```python
from build123d import *

# Parameters (mm, degrees)
BOSS_EXTRUDE1_DEPTH = 12
SKETCH2_R           = 5.25
CUT_EXTRUDE1_DEPTH  = 6
CHAMFER2_SIZE       = 3
CHAMFER2_SIZE2      = 5.196152423
SKETCH4_R           = 2.75
CUT_EXTRUDE3_DEPTH  = 28
CUT_EXTRUDE4_REACH  = 38.986
SKETCH5_W           = 8.2
SKETCH5_H           = 5.3
CUT_EXTRUDE6_REACH  = 38.986
CHAMFER3_SIZE       = 5
SKETCH8_R           = 2.95
BOSS_EXTRUDE2_DEPTH = 5
CHAMFER4_SIZE       = 5
CHAMFER4_SIZE2      = 10.722534603


with BuildPart() as part:
    # Sketch1 → Boss-Extrude1 (new, symmetric)
    with BuildSketch(Plane.XY):
        Polygon((-9, 8), (4, 8), (4, -30), (-14, -30), (-14, 0), (-3, 0), (-3, 4), (-9, 4), align=None)
    extrude(amount=BOSS_EXTRUDE1_DEPTH, both=True)

    # Sketch2 → Cut-Extrude1 (cut)
    with BuildSketch(Plane.XZ.offset(30)):
        with Locations((-5, 0)):
            Circle(SKETCH2_R)
    extrude(amount=-CUT_EXTRUDE1_DEPTH, mode=Mode.SUBTRACT)

    # Chamfer2
    chamfer2_edges = [part.edges().sort_by_distance(p)[0] for p in [
        (-14, 0, 0),
    ]]
    chamfer2_side = [part.faces().sort_by_distance(p)[0] for p in [
        (-8.5, 0, 0),
    ]]
    chamfer(chamfer2_edges, length=CHAMFER2_SIZE, length2=CHAMFER2_SIZE2, reference=chamfer2_side[0])

    # Sketch4 → Cut-Extrude3 (cut)
    with BuildSketch(Plane.XZ.offset(30)):
        with Locations((-5, 0)):
            Circle(SKETCH4_R)
    extrude(amount=-CUT_EXTRUDE3_DEPTH, mode=Mode.SUBTRACT)

    # Sketch5 → Cut-Extrude4 (cut, up to next)
    with BuildSketch(Plane(origin=(4, 0, 0), x_dir=(0, 0, -1), z_dir=(1, 0, 0)), mode=Mode.PRIVATE) as cut_extrude4_sk1:
        with Locations((0, -16.65)):
            Rectangle(SKETCH5_W, SKETCH5_H)
    cut_extrude4_tool1 = extrude(cut_extrude4_sk1.sketch, amount=-CUT_EXTRUDE4_REACH, mode=Mode.PRIVATE) & part.part
    add(cut_extrude4_tool1.solids().sort_by_distance((4, -16.65, 0))[0], mode=Mode.SUBTRACT)

    # Sketch7 → Cut-Extrude6 (cut, up to next)
    with BuildSketch(Plane(origin=(4, 0, 0), x_dir=(0, 0, -1), z_dir=(1, 0, 0)), mode=Mode.PRIVATE) as cut_extrude6_sk1:
        Polygon((-12, -30), (-12, -4), (-9, -8), (-9, -30), align=None)
    cut_extrude6_tool1 = extrude(cut_extrude6_sk1.sketch, amount=-CUT_EXTRUDE6_REACH, mode=Mode.PRIVATE) & part.part
    # Sketch7 → Cut-Extrude6 (cut, up to next)
    with BuildSketch(Plane(origin=(4, 0, 0), x_dir=(0, 0, -1), z_dir=(1, 0, 0)), mode=Mode.PRIVATE) as cut_extrude6_sk2:
        Polygon((9, -30), (12, -30), (12, -4), (9, -8), align=None)
    cut_extrude6_tool2 = extrude(cut_extrude6_sk2.sketch, amount=-CUT_EXTRUDE6_REACH, mode=Mode.PRIVATE) & part.part
    add(cut_extrude6_tool1.solids().sort_by_distance((4, -17.972222, 10.541667))[0], mode=Mode.SUBTRACT)
    add(cut_extrude6_tool2.solids().sort_by_distance((4, -17.972222, -10.541667))[0], mode=Mode.SUBTRACT)

    # Chamfer3
    # the kernel refuses this chamfer: 5 mm, written as the material it takes off along each edge
    with BuildSketch(Plane(origin=(4, 4.85841494, 9), x_dir=(0, 0, -1), z_dir=(0, -1, 0))) as chamfer3_piece_1_section:
        Polygon((CHAMFER3_SIZE, 0), (0, -CHAMFER3_SIZE), (0, 0), align=None)
    chamfer3_piece_1 = extrude(amount=47.71682988, mode=Mode.PRIVATE)
    chamfer3_piece_1 = split(chamfer3_piece_1, bisect_by=Plane(origin=(5.357524482, 4.043900251, 10.086019586), z_dir=(0.7071067811865478, -0.4242640687119279, 0.5656854249492383)), keep=Keep.TOP, mode=Mode.PRIVATE)
    add(chamfer3_piece_1, mode=Mode.SUBTRACT)
    with BuildSketch(Plane(origin=(4, 6.286731952, 19.715048964), x_dir=(0, 0.5999999999999992, -0.8000000000000004), z_dir=(0, -0.8000000000000005, -0.5999999999999993))) as chamfer3_piece_2_section:
        Polygon((CHAMFER3_SIZE, 0), (0, -CHAMFER3_SIZE), (0, 0), align=None)
    chamfer3_piece_2 = extrude(amount=30.71682988, mode=Mode.PRIVATE)
    chamfer3_piece_2 = split(chamfer3_piece_2, bisect_by=Plane(origin=(-3.857524482, 6.286731952, 11.857524482), z_dir=(0.7071067811865476, 0, 0.7071067811865476)), keep=Keep.TOP, mode=Mode.PRIVATE)
    add(chamfer3_piece_2, mode=Mode.SUBTRACT)
    with BuildSketch(Plane(origin=(4, 20.85841494, 12), x_dir=(0, 0, -1), z_dir=(0, -1, 0)), Plane(origin=(4, 20.85841494, -12), x_dir=(-1, 0, 0), z_dir=(0, -1, 0))) as chamfer3_piece_3:
        Polygon((CHAMFER3_SIZE, 0), (0, -CHAMFER3_SIZE), (0, 0), align=None)
    extrude(amount=37.71682988, mode=Mode.SUBTRACT)
    with BuildSketch(Plane(origin=(4, 6.286731952, -19.715048964), x_dir=(-1, 0, 0), z_dir=(0, -0.8000000000000006, 0.5999999999999993))) as chamfer3_piece_4_section:
        Polygon((CHAMFER3_SIZE, 0), (0, -CHAMFER3_SIZE), (0, 0), align=None)
    chamfer3_piece_4 = extrude(amount=30.71682988, mode=Mode.PRIVATE)
    chamfer3_piece_4 = split(chamfer3_piece_4, bisect_by=Plane(origin=(-3.857524482, 6.286731952, -11.857524482), z_dir=(0.7071067811865476, 0, -0.7071067811865476)), keep=Keep.TOP, mode=Mode.PRIVATE)
    add(chamfer3_piece_4, mode=Mode.SUBTRACT)
    with BuildSketch(Plane(origin=(4, 4.85841494, -9), x_dir=(0, 0, 1), z_dir=(0, -1, 0))) as chamfer3_piece_5_section:
        Polygon((CHAMFER3_SIZE, 0), (0, CHAMFER3_SIZE), (0, 0), align=None)
    chamfer3_piece_5 = extrude(amount=47.71682988, mode=Mode.PRIVATE)
    chamfer3_piece_5 = split(chamfer3_piece_5, bisect_by=Plane(origin=(5.357524482, 4.043900251, -10.086019586), z_dir=(0.7071067811865476, -0.424264068711928, -0.5656854249492386)), keep=Keep.TOP, mode=Mode.PRIVATE)
    add(chamfer3_piece_5, mode=Mode.SUBTRACT)
    with BuildSketch(Plane(origin=(-14, -42.85841494, -9), x_dir=(1, 0, 0), z_dir=(0, 1, 0))) as chamfer3_piece_6_section:
        Polygon((CHAMFER3_SIZE, 0), (0, -CHAMFER3_SIZE), (0, 0), align=None)
    chamfer3_piece_6 = extrude(amount=47.71682988, mode=Mode.PRIVATE)
    chamfer3_piece_6 = split(chamfer3_piece_6, bisect_by=Plane(origin=(-1.042475518, -35.083900251, 1.366019586), z_dir=(-0.7071067811865479, -0.42426406871192784, -0.5656854249492381)), keep=Keep.TOP, mode=Mode.PRIVATE)
    add(chamfer3_piece_6, mode=Mode.SUBTRACT)
    with BuildSketch(Plane(origin=(-14, -18.286731952, -1.284951036), x_dir=(1, 0, 0), z_dir=(0, 0.8000000000000006, -0.5999999999999993))) as chamfer3_piece_7_section:
        Polygon((CHAMFER3_SIZE, 0), (0, -CHAMFER3_SIZE), (0, 0), align=None)
    chamfer3_piece_7 = extrude(amount=29.221639351, mode=Mode.PRIVATE)
    chamfer3_piece_7 = split(chamfer3_piece_7, bisect_by=Plane(origin=(-15.357524482, -18.286731952, -2.642475518), z_dir=(-0.7071067811865476, 0, -0.7071067811865476)), keep=Keep.TOP, mode=Mode.PRIVATE)
    add(chamfer3_piece_7, mode=Mode.SUBTRACT)
    with BuildSketch(Plane(origin=(-4.57079253, 11.13571399, -12), x_dir=(0.8660254037844396, -0.49999999999999833, 0), z_dir=(-0.49999999999999833, -0.8660254037844397, 0))) as chamfer3_piece_8_section:
        Polygon((CHAMFER3_SIZE, 0), (0, CHAMFER3_SIZE), (0, 0), align=None)
    chamfer3_piece_8 = extrude(amount=30.335632033, mode=Mode.PRIVATE)
    chamfer3_piece_8 = split(chamfer3_piece_8, bisect_by=Plane(origin=(-4.57079253, 0, -12), z_dir=(0, -1, 0)), keep=Keep.TOP, mode=Mode.PRIVATE)
    add(chamfer3_piece_8, mode=Mode.SUBTRACT)
    with BuildSketch(Plane(origin=(-4.57079253, 11.13571399, 12), x_dir=(0, 0, -1), z_dir=(-0.49999999999999833, -0.8660254037844397, 0))) as chamfer3_piece_9_section:
        Polygon((CHAMFER3_SIZE, 0), (0, CHAMFER3_SIZE), (0, 0), align=None)
    chamfer3_piece_9 = extrude(amount=30.335632033, mode=Mode.PRIVATE)
    chamfer3_piece_9 = split(chamfer3_piece_9, bisect_by=Plane(origin=(-4.57079253, 0, 12), z_dir=(0, -1, 0)), keep=Keep.TOP, mode=Mode.PRIVATE)
    add(chamfer3_piece_9, mode=Mode.SUBTRACT)
    with BuildSketch(Plane(origin=(-14, -18.286731952, 1.284951036), x_dir=(0, 0.5999999999999993, -0.8000000000000005), z_dir=(0, 0.8000000000000005, 0.5999999999999993))) as chamfer3_piece_10_section:
        Polygon((CHAMFER3_SIZE, 0), (0, -CHAMFER3_SIZE), (0, 0), align=None)
    chamfer3_piece_10 = extrude(amount=29.221639351, mode=Mode.PRIVATE)
    chamfer3_piece_10 = split(chamfer3_piece_10, bisect_by=Plane(origin=(-15.357524482, -18.286731952, 2.642475518), z_dir=(-0.7071067811865476, 0, 0.7071067811865476)), keep=Keep.TOP, mode=Mode.PRIVATE)
    add(chamfer3_piece_10, mode=Mode.SUBTRACT)
    with BuildSketch(Plane(origin=(-14, -42.85841494, 9), x_dir=(0, 0, -1), z_dir=(0, 1, 0))) as chamfer3_piece_11_section:
        Polygon((CHAMFER3_SIZE, 0), (0, -CHAMFER3_SIZE), (0, 0), align=None)
    chamfer3_piece_11 = extrude(amount=47.71682988, mode=Mode.PRIVATE)
    chamfer3_piece_11 = split(chamfer3_piece_11, bisect_by=Plane(origin=(-1.042475518, -35.083900251, -1.366019586), z_dir=(-0.7071067811865476, -0.4242640687119281, 0.5656854249492385)), keep=Keep.TOP, mode=Mode.PRIVATE)
    add(chamfer3_piece_11, mode=Mode.SUBTRACT)

    # Sketch8 → Boss-Extrude2 (add)
    with BuildSketch(Plane.XZ.offset(30)):
        Polygon((4, 4), (-1, 9), (11, 9), (11, -9), (-1, -9), (4, -4), align=None)
        with Locations((7, 0)):
            Circle(SKETCH8_R, mode=Mode.SUBTRACT)
    extrude(amount=-BOSS_EXTRUDE2_DEPTH)

    # Chamfer4
    chamfer4_edges = [part.edges().sort_by_distance(p)[0] for p in [
        (11, -27.5, 9),
        (11, -27.5, -9),
    ]]
    chamfer4_side = [part.faces().sort_by_distance(p)[0] for p in [
        (11, -27.5, 0),
    ]]
    chamfer(chamfer4_edges, length=CHAMFER4_SIZE, length2=CHAMFER4_SIZE2, reference=chamfer4_side[0])


solid = part.part
```
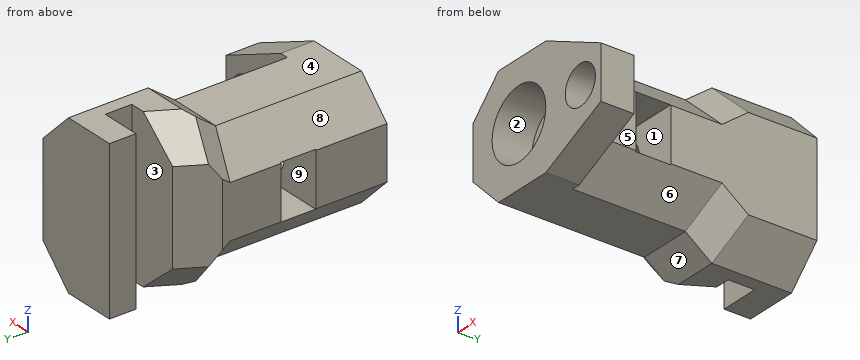
Can you work these out from the model? Positions are in its coordinate system, mm. Face numbers are marked on the shaded views. A direction names the side the tool comes from. Coordinates: 2 decimals unless noted, no trailing zeros. Loops run counter-clockwise (first coordinate to the right, second up) from the corner with the lowest first, then second, coordinate; pieces in that order, holes last. Notation, with made-up numbers: (-22.75, -2) -> (20.25, -2) arc R24 cw to (20.25, 35) -> close; hole circle Ø9 at (-24.5, -30). An arc over 180 degrees is marked (long way). Put each result on its own line as item: value. Start each with the question number.
Q1. I want a section at B-B (y = -8.5). Write out the boundary of the cut face in (x, z), plus the area to 3 significant figures.
Q2. If I drill on line 1 (Y direction, x = -7.5, z = 2.75); line 2 (Y direction, x = -1, z = -2.25); line 3 (Z direction, x = -5, y = -26.8), over which ranges is the centre line in solid material (lowest first)? Write a range as [from, to].
Q3. I want a section at D-D (x = 7). Write out the boundary of the cut face in (y, z).
Q4. I want a section at A-A (z = 0). Count the separate pieces of the cut face and the enclosed holes in it, plus the area to 3 significant figures.
Q5. Thinking about a two-plate mould opening in Y: for the marked faces 6, 7, 8 and 9, which applies, pulls with the +Y half, pulls with the -Y half, needs draft (parallel to the pull), parting line crosses it, or undercut?
Q6. I want a section at C-C (y = -26). Write out the boundary of the cut face in (x, z), plus the area to 3 significant figures.
Q7. I'm going to push flat-ended pins straight in: P1, Ø3, axis at y = -22, z = -1, coming from the +X side; P2, Ø1, axis at x = -3.5, y = -14, coming from the -Z side; P3, Ø6, axis at x = -5.5, z = -1, coming from the -Y side. Where does each tip first touch, or does it pass through?
Q8. For the marked faces 1, 2, 3, 4 and 5, which set-ups out of +Z, -Z, +X, -X, +Y, -Y let a thin tool reach every point of the face, with its end or its side?
Taken from the geometry:
1. outline: (-14, -4) -> (-9, -9) -> (-1, -9) -> (4, -4) -> (4, 4) -> (-1, 9) -> (-9, 9) -> (-14, 4) -> close; hole circle Ø5.5 at (-5, 0)
1. area: 250 mm2
2. line 1: y = [-24, -19.3], [-14, 0], [4, 8]
2. line 2: y = [-24, -19.3], [-14, 8]
2. line 3: z = [-9, -5.25], [5.25, 9]
3. outline: (-30, -5.87) -> (-25, -5.87) -> (-25, -2.95) -> (-30, -2.95) -> close; (-30, 2.95) -> (-25, 2.95) -> (-25, 5.87) -> (-30, 5.87) -> close
4. separate pieces: 4
4. enclosed holes: 0
4. area: 367 mm2
5. face 6: undercut
5. face 7: pulls with the -Y half
5. face 8: needs draft
5. face 9: undercut
6. outline: (-14, -4) -> (-9, -9) -> (0.28, -9) -> (11, -4) -> (11, 4) -> (0.28, 9) -> (-9, 9) -> (-14, 4) -> close; hole circle Ø10.5 at (-5, 0); hole circle Ø5.9 at (7, 0)
6. area: 257 mm2
7. P1: stops at x = 4
7. P2: stops at z = -9
7. P3: stops at y = -24
8. face 1: +X, -X
8. face 2: -Y
8. face 3: +Z, -Z, -X
8. face 4: +Z, +X, -X, -Y
8. face 5: +Z, -Z, +X, +Y
